Work out the finished part from the listing and answer in its coordinate system (mm). A direction names the side the tool comes from. Give positions to 0.01 mm unless a question says otherwise; leave off trailing zeros. Loops run counter-clockwise (first coordinate to the right, second up) from the corner with the lowest first, then second, coordinate; pieces in that order, holes last. Notation, with made-up numbers: (63, 10) - (97, 10) arc R13 cw to (97, 32) - close; hole circle Ø10 at (-40, -1.75). An arc over 180 degrees is marked (long way). One line per question, with ' | ' between items. Start each with the question number.
1. Each of these flat-tipped pins is pushed along its axis until it touches: pin 1 (5 mm diameter, centred on x = -10, y = 10, fed in from +Z); pin 2 (2 mm diameter, centred on y = 8, z = -2, fed in from -X). Where does it stop, or does it pass through?
2. Section C-C (y = 4.25) is taken. Determine the outline of the cut face in (x, z).
3. Section A-A (x = -6) is taken. Determine the outline of the cut face in (y, z).
4. Find the intervals of material crossed by line 1 (X direction, y = 4.5, z = -10); line 2 (X direction, y = 5.25, z = -11); line 3 (Z direction, x = -25, y = 5.5), in increasing order.
5. Section B-B (z = -10) is taken. Determine the outline of the cut face in (x, y).
6. Section D-D (y = 7.75) is taken. Determine the outline of the cut face in (x, z).
7. For a pull along X with two mould halves and no side action, classify faces 3 (the face through (-18.67, 11.625, -11.406)), 4 (the face through (-14, 3, -20)), 5 (the face through (-0.86, 3.04, -19.1)), 6 (the face through (-8.5, 3, -10)) as released by +X, released by -X, zero draft, split by the parting line, or undercut.
8. Which of the six approach directions +Z, -Z, +X, -X, +Y, -Y give full straight-line access (tool end or side, diameter ignored) to faces 1 (the face through (-0.9, 3.04, -0.86)), 2 (the face through (-5.95, 3.04, -3.75))?
from build123d import *

# Parameters (mm, degrees)
Y_KSEKLIK_EKSTR_ZYON1_DEPTH = 6
IZIM2_R                     = 6.25
IZIM2_R_2                   = 3.75
Y_KSEKLIK_EKSTR_ZYON2_DEPTH = 6
KES_EKSTR_ZYON1_DEPTH       = 6
IZIM5_R                     = 3.75
KES_EKSTR_ZYON2_DEPTH       = 6
RADYUS1_R                   = 3
RADYUS2_R                   = 3


with BuildPart() as part:
    # Çizim1 → Yükseklik-Ekstrüzyon1 (new body)
    with BuildSketch(Plane(origin=(0, 0, 0), x_dir=(1, 0, 0), z_dir=(0, 1, 0))):
        with BuildLine():
            ThreePointArc((-25, 20), (-35, 10), (-25, 0))
            Line((-25, 0), (-25, 20))
        make_face()
        with BuildLine():
            Line((-25, 20), (-25, 0))
            ThreePointArc((-25, 0), (-17.928932188, 2.928932188), (-15, 10))
            ThreePointArc((-15, 10), (-17.928932188, 17.071067812), (-25, 20))
        make_face()
        with BuildLine():
            Line((-25, 0), (0, 0))
            Line((0, 0), (0, 20))
            Line((0, 20), (-25, 20))
            ThreePointArc((-25, 20), (-17.928932188, 17.071067812), (-15, 10))
            ThreePointArc((-15, 10), (-17.928932188, 2.928932188), (-25, 0))
        make_face()
    extrude(amount=Y_KSEKLIK_EKSTR_ZYON1_DEPTH)

    # Çizim2 → Yükseklik-Ekstrüzyon2 (add)
    with BuildSketch(Plane(origin=(0, 6, 0), x_dir=(1, 0, 0), z_dir=(0, 1, 0))):
        with Locations((-25, 10)):
            Circle(IZIM2_R)
        with Locations((-25, 10)):
            Circle(IZIM2_R_2, mode=Mode.SUBTRACT)
    extrude(amount=Y_KSEKLIK_EKSTR_ZYON2_DEPTH)

    # Çizim4 → Kes-Ekstrüzyon1 (cut)
    with BuildSketch(Plane(origin=(0, 6, 0), x_dir=(1, 0, 0), z_dir=(0, 1, 0))):
        with BuildLine():
            Line((-3.5, 13.75), (-3.5, 6.25))
            ThreePointArc((-3.5, 6.25), (-6, 3.75), (-8.5, 6.25))
            Line((-8.5, 6.25), (-8.5, 13.75))
            ThreePointArc((-8.5, 13.75), (-6, 16.25), (-3.5, 13.75))
        make_face()
    extrude(amount=-KES_EKSTR_ZYON1_DEPTH, mode=Mode.SUBTRACT)

    # Çizim5 → Kes-Ekstrüzyon2 (cut)
    with BuildSketch(Plane(origin=(0, 6, 0), x_dir=(1, 0, 0), z_dir=(0, 1, 0))):
        with Locations((-25, 10)):
            Circle(IZIM5_R)
    extrude(amount=-KES_EKSTR_ZYON2_DEPTH, mode=Mode.SUBTRACT)

    # Radyus1
    radyus1_edges = [part.edges().sort_by_distance(p)[0] for p in [
        (0, 3, 0),
    ]]
    fillet(radyus1_edges, radius=RADYUS1_R)

    # Radyus2
    radyus2_edges = [part.edges().sort_by_distance(p)[0] for p in [
        (0, 3, -20),
    ]]
    fillet(radyus2_edges, radius=RADYUS2_R)

    # Çizim6 → Döndür1 (revolve)
    with BuildSketch(Plane(origin=(-25, 0, 0), x_dir=(0, 0, -1), z_dir=(1, 0, 0))):
        Polygon((3.75, 12), (0, 6), (3.75, 6), align=None)
    revolve(axis=Axis((-25, 12, -10), (0, -1, 0)))


solid = part.part
Conclusion:
1) pin 1: through | pin 2: x = -30.61
2) outline: (-25, -20) - (-3, -20) arc R3 ccw to (0, -17) - (0, -3) arc R3 ccw to (-3, 0) - (-25, 0) arc R10 ccw to start; hole circle Ø7.5 at (-25, -10); hole (-8.5, -13.75) arc R2.5 ccw to (-3.5, -13.75) - (-3.5, -6.25) arc R2.5 ccw to (-8.5, -6.25) - close
3) outline: (0, -20) - (6, -20) - (6, -16.25) - (0, -16.25) - close; (0, -3.75) - (6, -3.75) - (6, 0) - (0, 0) - close
4) line 1: -35 to -28.75, -21.25 to -8.5, -3.5 to 0 | line 2: -34.95 to -28.61, -21.39 to -8.5, -3.5 to 0 | line 3: -20 to -13.75, -6.25 to 0
5) outline: (-35, 0) - (-28.75, 0) - (-28.75, 12) - (-31.25, 12) - (-35, 6) - close; (-21.25, 0) - (-8.5, 0) - (-8.5, 6) - (-15, 6) - (-18.75, 12) - (-21.25, 12) - close; (-3.5, 0) - (0, 0) - (0, 6) - (-3.5, 6) - close
6) outline: circle Ø17.81 at (-25, -10); hole circle Ø7.5 at (-25, -10)
7) face 3: split by the parting line | face 4: zero draft | face 5: released by +X | face 6: undercut
8) face 1: +Z, +X, +Y, -Y | face 2: +Y, -Y
